The model under review builds one solid part; all positions refer to its coordinate system, in mm. Face numbers are marked on the shaded views. A direction names the side the tool comes from. Round coordinates to 2 decimals unless told otherwise and drop trailing zeros. Write each loop counter-clockwise with the first axis right and the second up, starting at its lowest first coordinate (ties: lowest second). Pieces come first, ordered by that corner, then holes.
Item 1: Clearance check with a flat-ended pin moving along its axis: pin 1 Ø22 at (x, y) = (-2, 2) entering from +Z. State where the tip first meets the part, or that it passes through.
Item 2: Add section A-A (z = 73). Give the boundary of the cut face in (x, y), plus the area to 3 significant figures.
Item 3: Draft analysis for pull direction Y (two halves, no side actions). For the marked faces 3, 4 and 5, state which applies: +Y half, -Y half, draft (parallel to the pull), parting line (faces both ways), or undercut.
Item 4: Add section D-D (x = 0). Give the boundary of the cut face in (y, z), plus the area to 3 significant figures.
Item 5: Add section C-C (y = 0). Give the boundary of the cut face in (x, z), plus the area to 3 significant figures.
Item 6: To check wall thickness, follow L1, parallel to Y at x = 0, z = 65; L2, parallel to Z at x = -12, y = 27.5; L3, parallel to Z at x = 9.5, y = -2. State the ranges of each line that lie inside material, in increasing order.
Item 7: Add section B-B (x = 40). Give the boundary of the cut face in (y, z), plus the area to 3 significant figures.
Item 8: Machinability: for the marked faces 1 and 2, which of the approach directions +Z, -Z, +X, -X, +Y, -Y give a long, thin tool a straight path to every point of the face, cutting with its end or side? Answer none if there is none.
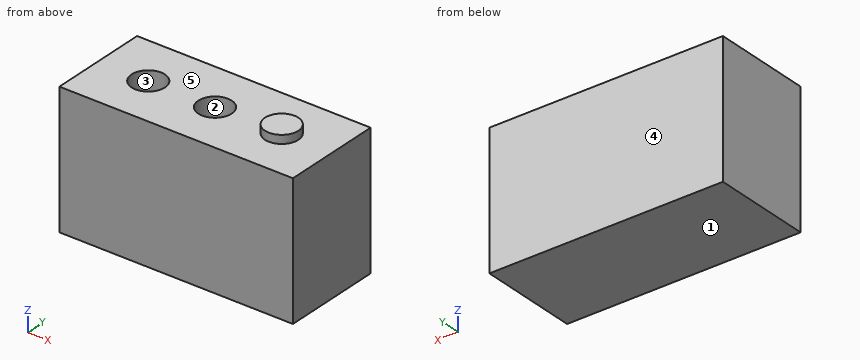
```python
from build123d import *

# Parameters (mm, degrees)
F0_W     = 140
F0_H     = 60
F1_DEPTH = 60
F2_W     = 140
F2_H     = 60
F2_R     = 10
F5_DEPTH = 20
F4_R     = 10
F8_DEPTH = 500
F3_R     = 10
F9_DEPTH = 25


with BuildPart() as f1:
    # F0 (on Top) → F1 (new body)
    with BuildSketch(Plane.XY):
        Rectangle(F0_W, F0_H)
    extrude(amount=F1_DEPTH)

    # F2 (on face) → F5 (join)
    with BuildSketch(Plane.XY.offset(60)):
        Rectangle(F2_W, F2_H)
        with Locations((-40, 0)):
            Circle(F2_R, mode=Mode.SUBTRACT)
    extrude(amount=F5_DEPTH)

    # F4 (on face) → F8 (cut)
    with BuildSketch(Plane.XY.offset(60)):
        Circle(F4_R)
    extrude(amount=F8_DEPTH, mode=Mode.SUBTRACT)

    # F3 (on face) → F9 (join)
    with BuildSketch(Plane.XY.offset(60)):
        with Locations((40, 0)):
            Circle(F3_R)
    extrude(amount=F9_DEPTH)


solid = f1.part
```
Numbers:
1. pin 1: stops at z = 80
2. outline: (-70, -30) - (70, -30) - (70, 30) - (-70, 30) - close; hole circle Ø20 at (-40, 0); hole circle Ø20 at (0, 0)
2. area: 7,770 mm2
3. face 3: undercut
3. face 4: +Y half
3. face 5: draft
4. outline: (-30, 0) - (30, 0) - (30, 80) - (10, 80) - (10, 60) - (-10, 60) - (-10, 80) - (-30, 80) - close
4. area: 4,400 mm2
5. outline: (-70, 0) - (70, 0) - (70, 80) - (50, 80) - (50, 85) - (30, 85) - (30, 80) - (10, 80) - (10, 60) - (-10, 60) - (-10, 80) - (-30, 80) - (-30, 60) - (-50, 60) - (-50, 80) - (-70, 80) - close
5. area: 10,500 mm2
6. L1: y = -30 to -10, 10 to 30
6. L2: z = 0 to 80
6. L3: z = 0 to 60
7. outline: (-30, 0) - (30, 0) - (30, 80) - (10, 80) - (10, 85) - (-10, 85) - (-10, 80) - (-30, 80) - close
7. area: 4,900 mm2
8. face 1: -Z, +X, -X, +Y, -Y
8. face 2: +Z
